```python
from build123d import *

# Parameters (mm, degrees)
CUT_EXTRUDE1_START = 1.245
CUT_EXTRUDE1_DEPTH = 7.37
CIRPATTERN1_COUNT  = 12
SKETCH4_R          = 1.4224
CUT_EXTRUDE2_DEPTH = 12.190650428
CUT_EXTRUDE3_DEPTH = 1.0668
CHAMFER1_SIZE      = 0.28075


with BuildPart() as part:
    # Sketch2 → Revolve1 (revolve)
    with BuildSketch(Plane(origin=(0, 0, 0), x_dir=(0, 0, -1), z_dir=(1, 0, 0)), mode=Mode.PRIVATE) as revolve1_sk:
        Polygon((-7.135, 1.5875), (7.135, 1.5875), (7.135, 6.096), (6.63, 6.096), (6.125, 4.83225), (6.125, 3.5685), (-1.245, 3.5685), (-1.245, 4.83225), (-1.75, 6.096), (-7.135, 6.096), align=None)
    revolve(revolve1_sk.sketch.rotate(Axis((0, 0, 7.135), (0, 0, -1)), 90), axis=Axis((0, 0, 7.135), (0, 0, -1)))

    # Sketch3 → Cut-Extrude1 (cut)
    with BuildSketch(Plane.XY.offset(CUT_EXTRUDE1_START)):
        with BuildLine():
            Line((3.566654882, 6.096), (-3.566654882, 6.096))
            Line((-3.566654882, 6.096), (-1.802078902, 3.080049331))
            ThreePointArc((-1.802078902, 3.080049331), (-1.296607682, 3.324605355), (-0.759031417, 3.486841487))
            ThreePointArc((-0.759031417, 3.486841487), (-0.645131247, 3.465879975), (-0.580109509, 3.370042573))
            ThreePointArc((-0.580109509, 3.370042573), (-0.547109503, 3.247589437), (-0.498876404, 3.130297753))
            ThreePointArc((-0.498876404, 3.130297753), (0, 2.8185), (0.498876404, 3.130297753))
            ThreePointArc((0.498876404, 3.130297753), (0.547109503, 3.247589437), (0.580109509, 3.370042573))
            ThreePointArc((0.580109509, 3.370042573), (0.645131247, 3.465879975), (0.759031417, 3.486841487))
            ThreePointArc((0.759031417, 3.486841487), (1.296607682, 3.324605355), (1.802078902, 3.080049331))
            Line((1.802078902, 3.080049331), (3.566654882, 6.096))
        make_face()
    cut_extrude1 = extrude(amount=-CUT_EXTRUDE1_DEPTH, mode=Mode.SUBTRACT)

    # CirPattern1: Cut-Extrude1 ×12 about axis
    cirpattern1_axis = Axis((0, 0, 0), (0, 0, 1))
    for i in range(1, CIRPATTERN1_COUNT):
        add(cut_extrude1.rotate(cirpattern1_axis, i * 360 / CIRPATTERN1_COUNT), mode=Mode.SUBTRACT)

    # Sketch4 → Cut-Extrude2 (cut, through all)
    with BuildSketch(Plane(origin=(0, 0, 0), x_dir=(0, -1, 0), z_dir=(1, 0, 0))):
        with Locations(Location((0, -4.19, 0), (0, 0, 270))):
            Circle(SKETCH4_R)
    extrude(amount=CUT_EXTRUDE2_DEPTH, mode=Mode.SUBTRACT)

    # Sketch5 → Revolve2 (revolve)
    with BuildSketch(Plane.XY.offset(4.19), mode=Mode.PRIVATE) as revolve2_sk:
        Polygon((1.5875, -1.0414), (1.5875, 0), (5.927730952, 0), (5.927730952, -1.0414), (5.546730952, -1.4224), (1.9685, -1.4224), align=None)
    revolve(revolve2_sk.sketch.rotate(Axis((1.5875, 0, 4.19), (1, 0, 0)), 270), axis=Axis((1.5875, 0, 4.19), (1, 0, 0)))

    # Sketch6 → Cut-Extrude3 (cut)
    with BuildSketch(Plane(origin=(5.927730952, 5.384140679, 0), x_dir=(0, -1, 0), z_dir=(-1, 0, 0))):
        Polygon((5.384140679, 5.011223023), (4.672940679, 4.600611511), (4.672940679, 3.779388489), (5.384140679, 3.368776977), (6.095340679, 3.779388489), (6.095340679, 4.600611511), align=None)
    extrude(amount=CUT_EXTRUDE3_DEPTH, mode=Mode.SUBTRACT)

    # Chamfer1
    chamfer1_edges = [part.edges().sort_by_distance(p)[0] for p in [
        (-1.5875, 0, 7.135),
        (-6.096, 0, 7.135),
    ]]
    chamfer(chamfer1_edges, length=CHAMFER1_SIZE)


solid = part.part
```
Work out the finished part from the listing and answer in its coordinate system (mm). A direction names the side the tool comes from. Give positions to 0.01 mm unless a question says otherwise; leave off trailing zeros. Answer as CSV lines item,"result". Start each with the question number.
(1) For a pull along X with two mould halves and no side action, classify faces 1 (the flat face through (5.4, 0.711, 4.2)), 2 (the cylindrical face through (-0.01, 2.82, -2.39)), 3 (the cylindrical face through (-2.82, -0.01, -2.39)) as released by +X, released by -X, zero draft, split by the parting line, or undercut.
(2) Which of the six approach directions +Z, -Z, +X, -X, +Y, -Y give full straight-line access (tool end or side, diameter ignored) to faces 4 (the flat face through (5.4, -0.711, 4.2)), 5 (the flat face through (-1.3, 1.3, -7.135)), 6 (the cylindrical face through (2.437, 1.417, -2.388)), 7 (the cylindrical face through (0.01, -2.82, -2.39))?
(3) Consider line 1 along Z through (x, y) = (2, 3.75) (3 decimals); line 2 along X through (y, z) = (2.5, -0.25); line 3 along X through (y, z) = (-3.25, -1.75). Determine where each line is inside the solid, lowest interval first.
(4) Each of these flat-tipped pins is pushed along its axis until it touches: pin 1 Ø2 at (y, z) = (2, -3) entering from -X; pin 2 Ø1.9 at (x, y) = (0, 0) entering from -Z; pin 3 Ø0.9 at (x, z) = (5, 4.5) entering from -Y; pin 4 Ø5 at (x, y) = (0.5, 1) entering from +Z (3 decimals). Where does it stop, or does it pass through?
Entries:
1,face 1,"zero draft"
1,face 2,"undercut"
1,face 3,"released by -X"
2,face 4,"+X"
2,face 5,"-Z, +X, -X, +Y, -Y"
2,face 6,"none"
2,face 7,"-Y"
3,line 1,"-7.135 to -6.125, 1.245 to 7.135"
3,line 2,"-2.55 to -2.05, -1.33 to 1.33, 2.05 to 2.55"
3,line 3,"-1.19 to -0.55, 0.55 to 1.19"
4,pin 1,"x = -3.43"
4,pin 2,"through"
4,pin 3,"y = -4.06"
4,pin 4,"z = 7.135"
